Source: CAD feature listing. Evaluate the final solid. Frame: model axes, mm. Face numbers are marked on the shaded views. A direction names the side the tool comes from. Round coordinates to 2 decimals unless told otherwise and drop trailing zeros. Loops run counter-clockwise (first coordinate to the right, second up) from the corner with the lowest first, then second, coordinate; pieces in that order, holes last.
(1) Section A-A, the plane x = 0. Return the cut outline in (y, z).
(2) Set-up query: the marked faces 1 and 2. Return all of +Z, -Z, +X, -X, +Y, -Y with unobstructed straight access to the full face (end or side cutting, diameter ignored); none if empty.
(3) First-contact query: pin 1 Ø6 at (y, z) = (1, 8.5) entering from +X; pin 2 Ø3.5 at (x, y) = (0, 8) entering from -Z; pin 3 Ø4 at (x, z) = (2.5, 4.5) entering from -Y; pin 4 Ø2.5 at (x, y) = (8, 0) entering from +Z. Flat tips, straight axial feed; report the tip coordinate or a pass-through.
(4) Section B-B, the plane y = -8. Return the cut outline in (x, z), plus the area to 3 significant figures.
(5) Section D-D, the plane x = 7.5. Return the cut outline in (y, z).
(6) Material intervals for probe 1 along Y at (x, z) = (0, 0.9); probe 2 along Y at (x, z) = (0, 3.25); probe 3 along Z at (x, y) = (7.5, -2.5), sorted ascending.
(7) Mould query, pull axis Y, two halves, no side actions, for the marked faces 3, 4 and 5. Classes: pulls with the +Y half, pulls with the -Y half, needs draft (parallel to the pull), parting line crosses it, or undercut.
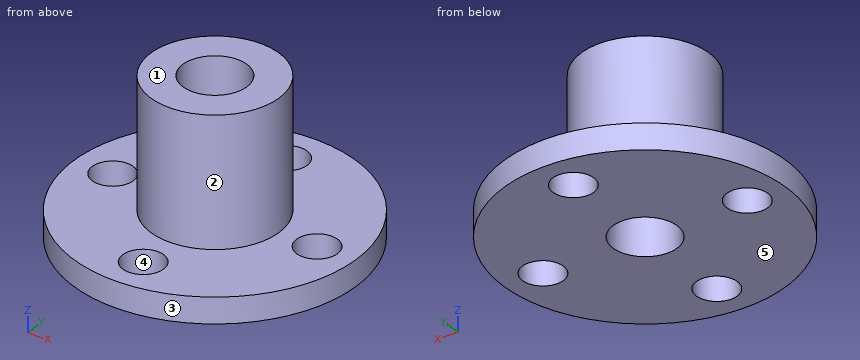
```python
from build123d import *

# Parameters (mm, degrees)
SKETCH_1_R                  = 11
EXTRUDE_1_DEPTH             = 2
SKETCH_2_R                  = 5
EXTRUDE_2_DEPTH             = 10
SKETCH_3_R                  = 2.5
CUT_EXTRUDE_1_DEPTH         = 20.646882704
HOLE_WIZARD_3_2_3_2_1_D     = 3.2
HOLE_WIZARD_3_2_3_2_1_DEPTH = 10
HOLE_WIZARD_3_2_3_2_1_TIP   = 0.96137699


with BuildPart() as part:
    # 草图1 → 凸台-拉伸1 (new body)
    with BuildSketch(Plane.XY):
        Circle(SKETCH_1_R)
    extrude(amount=EXTRUDE_1_DEPTH)

    # 草图2 → 凸台-拉伸2 (add)
    with BuildSketch(Plane.XY.offset(2)):
        Circle(SKETCH_2_R)
    extrude(amount=EXTRUDE_2_DEPTH)

    # 草图3 → 切除-拉伸1 (cut, through all)
    with BuildSketch(Plane.XY.offset(12)):
        Circle(SKETCH_3_R)
    extrude(amount=-CUT_EXTRUDE_1_DEPTH, mode=Mode.SUBTRACT)

    # Ø3.2 (3.2) 直径孔1
    with Locations(Plane.XY.offset(2)):
        with Locations((8, 0), (-8, 0), (0, -8), (0, 8)):
            Hole(HOLE_WIZARD_3_2_3_2_1_D / 2, depth=HOLE_WIZARD_3_2_3_2_1_DEPTH)
            with Locations((0, 0, -(HOLE_WIZARD_3_2_3_2_1_DEPTH + HOLE_WIZARD_3_2_3_2_1_TIP / 2))):  # 118° drill point
                Cone(0, HOLE_WIZARD_3_2_3_2_1_D / 2, HOLE_WIZARD_3_2_3_2_1_TIP, mode=Mode.SUBTRACT)


solid = part.part
```
Output values:
1. outline: (-11, 0) - (-9.6, 0) - (-9.6, 2) - (-11, 2) - close; (-6.4, 0) - (-2.5, 0) - (-2.5, 12) - (-5, 12) - (-5, 2) - (-6.4, 2) - close; (2.5, 0) - (6.4, 0) - (6.4, 2) - (5, 2) - (5, 12) - (2.5, 12) - close; (9.6, 0) - (11, 0) - (11, 2) - (9.6, 2) - close
2. face 1: +Z, +X, -X, +Y, -Y
2. face 2: +Z
3. pin 1: stops at x = 5
3. pin 2: stops at z = 0
3. pin 3: stops at y = -4.97
3. pin 4: passes through
4. outline: (-7.55, 0) - (-1.6, 0) - (-1.6, 2) - (-7.55, 2) - close; (1.6, 0) - (7.55, 0) - (7.55, 2) - (1.6, 2) - close
4. area: 23.8 mm2
5. outline: (-8.05, 0) - (-1.52, 0) - (-1.52, 2) - (-8.05, 2) - close; (1.52, 0) - (8.05, 0) - (8.05, 2) - (1.52, 2) - close
6. probe 1: y = -11 to -9.6, -6.4 to -2.5, 2.5 to 6.4, 9.6 to 11
6. probe 2: y = -5 to -2.5, 2.5 to 5
6. probe 3: z = 0 to 2
7. face 3: parting line crosses it
7. face 4: undercut
7. face 5: needs draft
